```python
from build123d import *

# Parameters (mm, degrees)
F1_DEPTH    = 35
F2_T1_DEPTH = 55


# Not quite as in the source:
# - a fillet or chamfer that OpenCascade refuses, or shapes differently, is made with other operations: its cross-section is extruded or revolved along the edge and cut away or added


with BuildPart() as f1:
    # F0 (on Front) → F1 (new body)
    with BuildSketch(Plane.XZ):
        with BuildLine():
            Line((-15.5290191181, 81.5544475097), (-17.315076228, 80.6544475097))
            Line((-17.315076228, 80.6544475097), (12.2598850951, 21.9627031234))
            ThreePointArc((12.2598850951, 21.9627031234), (11.4910392166, 3.9362212778), (-4.2611431719, -4.8622968766))
            Line((-4.2611431719, -4.8622968766), (-45.5504947187, -4.8622968766))
            ThreePointArc((-45.5504947187, -4.8622968766), (-61.3026771072, 3.9362212778), (-62.0715229858, 21.9627031234))
            Line((-62.0715229858, 21.9627031234), (-32.4965616626, 80.6544475097))
            Line((-32.4965616626, 80.6544475097), (-34.2826187726, 81.5544475097))
            Line((-34.2826187726, 81.5544475097), (-63.8575800957, 22.8627031234))
            ThreePointArc((-63.8575800957, 22.8627031234), (-63.0056157438, 2.8874124296), (-45.5504947187, -6.8622968766))
            Line((-45.5504947187, -6.8622968766), (-4.2611431719, -6.8622968766))
            ThreePointArc((-4.2611431719, -6.8622968766), (13.1939778532, 2.8874124296), (14.0459422051, 22.8627031234))
            Line((14.0459422051, 22.8627031234), (-15.5290191181, 81.5544475097))
        make_face()
    extrude(amount=F1_DEPTH)

    # F2: fillet of radius 5 on 2 edges, made by hand

    # F2_s2 → F2_t1 (cut)
    with BuildSketch(Plane.XZ.offset(-10)):
        with BuildLine():
            ThreePointArc((-34.2965616626, 77.0823332898), (-33.7617287381, 79.3167446648), (-34.2826187726, 81.5544475097))
            Line((-34.2826187726, 81.5544475097), (-32.4965616626, 80.6544475097))
            Line((-32.4965616626, 80.6544475097), (-34.2965616626, 77.0823332898))
        make_face()
        with BuildLine():
            ThreePointArc((-15.5290191181, 81.5544475097), (-16.0499091526, 79.3167446648), (-15.515076228, 77.0823332898))
            Line((-15.515076228, 77.0823332898), (-17.315076228, 80.6544475097))
            Line((-17.315076228, 80.6544475097), (-15.5290191181, 81.5544475097))
        make_face()
    extrude(amount=F2_T1_DEPTH, mode=Mode.SUBTRACT)


solid = f1.part
```
CAD build for the part. Positions are in the model's coordinates, mm. A direction names the side the tool comes from. Round coordinates to 2 decimals unless told otherwise and drop trailing zeros. Loops run counter-clockwise (first coordinate to the right, second up) from the corner with the lowest first, then second, coordinate; pieces in that order, holes last. Notation, with made-up numbers: M -3.75,36.25 L 43.25,36.25 A26 cw 43.25,62.25 Z; hole C 25.5,-26.75 d3. An arc over 180 degrees is marked long. Use a Markdown table: item, result. Add a question column.
(1) Pull direction Z, two halves, no side cores. Call faces 1 (the face through (-61.16, -17.26, 3.71)), 2 (the face through (-48.863, -17.255, 52.619)), 3 (the face through (-25.1, -35, -5.02)): +Z half, -Z half, draft (parallel to the pull), parting line (faces both ways), or undercut.
(2) Cut at C-C (y = -20). Give the cut face in (x, z), and give its area (3 significant figures).
(3) Flat gauge pins, fed straight in: pin 1 (2 mm diameter, centred on x = 2.5, z = 45, fed in from +Y); pin 2 (2 mm diameter, centred on y = -16.5, z = 65.5, fed in from +X); pin 3 (2 mm diameter, centred on y = -10, z = 8.5, fed in from +X). Where does each tip first touch, or does it go through?
(4) Cut at A-A (x = 11). Give the cut face in (y, z), and give its area (3 significant figures).
(5) Cut at B-B (z = 67.5). Give the cut face in (x, y).
(6) Cut at D-D (x = -18.5). Give the cut face in (y, z).
(7) Which spindle directions (+Z, -Z, +X, -X, +Y, -Y) get a long thin tool onto all of the face, cutting with end or side? Do faces 4 (the face through (-63.16, -17.26, 3.14)), 5 (the face through (-48.378, -17.255, 49.137)). Say none if no direction does.
(8) Drill centre lines: line 1 (Z direction, x = 9, y = -13.5); line 2 (Z direction, x = -5.5, y = -24.5); line 3 (Z direction, x = -17.5, y = -27). Where is each one in solid material? Low to high.
Geometry says:
| question | item | result |
|---|---|---|
| 1 | face 1 | undercut |
| 1 | face 2 | +Z half |
| 1 | face 3 | draft |
| 2 | outline | M -63.86,22.86 A20.5 ccw -45.55,-6.86 L -4.26,-6.86 A20.5 ccw 14.05,22.86 L -15.53,81.55 A5 ccw -15.52,77.08 L 12.26,21.96 A18.5 cw -4.26,-4.86 L -45.55,-4.86 A18.5 cw -62.07,21.96 L -34.3,77.08 A5 ccw -34.28,81.55 Z |
| 2 | area | 500 mm² |
| 3 | pin 1 | stops at y = 0 |
| 3 | pin 2 | stops at x = -6.94 |
| 3 | pin 3 | stops at x = 15.82 |
| 4 | outline | M -35,-0.05 L 0,-0.05 L 0,3.18 L -35,3.18 Z; M -35,24.46 L 0,24.46 L 0,28.91 L -35,28.91 Z |
| 4 | area | 269 mm² |
| 5 | outline | M -41.36,-35 L -39.13,-35 L -39.13,0 L -41.36,0 Z; M -10.69,-35 L -8.45,-35 L -8.45,0 L -10.69,0 Z |
| 6 | outline | M -35,-6.86 L 0,-6.86 L 0,-4.86 L -35,-4.86 Z |
| 7 | face 4 | -X, +Y, -Y |
| 7 | face 5 | +Y, -Y |
| 8 | line 1 | z = -2 to 0.74, 28.43 to 32.88 |
| 8 | line 2 | z = -6.86 to -4.86, 57.21 to 61.65 |
| 8 | line 3 | z = -6.86 to -4.86 |
